Autodesk Inventor part; units mm, degrees
ref_plane "Work Plane1" through (0, 0, 0) normal (0, -0.9396926, -0.3420201) x (-1, 0, 0)
ref_plane "YZ Plane" through (0, 0, 0) normal (1, 0, 0) x (0, 1, 0)
ref_plane "XZ Plane" through (0, 0, 0) normal (0, 1, 0) x (-1, 0, 0)
sketch "Sketch2" plane through (0, 0, 0) normal (0, 1, 0) x (-1, 0, 0)
  line L0 (0, 0) -> (-7, 0)
  line L1 (-7, 0) -> (-7, -10)
  line L2 (-7, -10) -> (0, -10)
  line L3 (0, -10) -> (0, 0)
  circle A0 centre (-3.5, -5) radius 1.65
  line L4 (0, 0) -> (15, 0)
  line L5 (15, 0) -> (15, -15.9854)
  line L6 (15, -15.9854) -> (0, -15.9854)
  line L7 (0, -15.9854) -> (0, 0)
  line L8 (7.8, 0) -> (10.8, 0)
  line L9 (10.8, 0) -> (10.8, -15.9854)
  line L10 (10.8, -15.9854) -> (7.8, -15.9854)
  line L11 (7.8, -15.9854) -> (7.8, 0)
  line L12 (15, -15.9854) -> (10.8, -15.9854)
  line L13 (10.8, -15.9854) -> (10.8, -4.2527)
  line L14 (10.8, -4.2527) -> (15, -4.2527)
  line L15 (15, -4.2527) -> (15, -15.9854)
  line L16 (0, -10) -> (10.8, -10)
  point P0 (0, -5)
  point P1 (-3.5, -10)
  point P2 (10.8, 0)
  point P3 (15, -4.2527)
  point P4 (7.8, -10)
  dimension "d2" = 7
  dimension "d3" = 10
  dimension "d4" = 3.3
  dimension "d12" = 22
  dimension "d21" = 11.3
  dimension "d22" = 3
extrude "Extrusion1" add sketch "Sketch2" along normal blind 4.5 contours L3 L2 L1 L0
extrude "Extrusion2" add sketch "Sketch2" along normal blind 4 contours L4 L11 L16 L3 | L4 L9 L16 L11 | L4 L5 L14 L9
ref_plane "Work Plane1" through (0, 0, 0) normal (0, -0.9396926, -0.3420201) x (-1, 0, 0)
sketch "Sketch4" plane through (-15, 0, -15.9854) normal (-1, 0, 0) x (0, 0, 1)
  line L0 (-0.8784, 3) -> (12.8006, -3.1551)
  line L1 (12.8006, -3.1551) -> (13.2109, -2.2432)
  line L2 (13.2109, -2.2432) -> (-0.4681, 3.9119)
  line L3 (-0.8784, 3) -> (-0.4681, 3.9119)
  arc A0 (18.4229, -40.6351) -> (9.5813, -1.7065) centre (-0.6772, -24.5048) ccw
  line L4 (18.4229, -40.6351) -> (19.1869, -41.2803)
  line L5 (9.5813, -1.7065) -> (10.2986, -0.9327)
  arc A1 (19.1869, -41.2803) -> (10.2986, -0.9327) centre (-0.2668, -24.413) ccw
  arc A2 (18.4229, -40.6351) -> (17.1504, -48.2979) centre (24.2261, -45.5359) ccw
  arc A3 (19.1869, -41.2803) -> (18.0819, -47.9342) centre (24.064, -45.509) ccw
  line L6 (17.1504, -48.2979) -> (18.0819, -47.9342)
  line L7 (22.6596, -12.694) -> (22.6596, 0.6055)
  line L8 (22.6596, 0.6055) -> (12.4332, 0.6055)
  line L9 (12.4332, 0.6055) -> (12.4332, 1.6055)
  line L10 (12.4332, 1.6055) -> (23.6596, 1.6055)
  line L11 (23.6596, 1.6055) -> (23.6596, -14.9008)
  line L12 (5.9854, 0) -> (11.7327, 0)
  arc A4 (2.815, 4.6033) -> (3.1019, 1.209) centre (3.9014, 2.9858) ccw
  line L13 (2.815, 4.6033) -> (2.815, 3.6033)
  arc A5 (2.815, 3.6033) -> (3.0226, 2.3412) centre (3.3375, 3.0411) ccw
  point P0 (15.9854, 0)
  point P1 (13.4215, -1.7995)
  point P2 (1.9601, 2.8193)
  point P3 (2.654, 2.6401)
  dimension "d14" = 1
  dimension "d20" = 15
  dimension "d26" = 25
  dimension "d27" = 1
  dimension "d29" = 1
  dimension "d30" = 1
  dimension "d31" = 1
  dimension "d35" = 3
  dimension "d37" = 1
  dimension "d38" = 1
extrude "Extrusion4" add sketch "Sketch4" along normal blind 10 contours A4 L2 L5 L0 | L5 A1 L1 L0 | L0 L1 A1 L4 A0 | A4 L13 A5 L2 | L4 A3 L6 A2 | L7 L8 L9 L10 L11 A1
extrude "Extrusion5" add sketch "Sketch2" against normal blind 6 contours L4 L9 L16 L11
chamfer "Chamfer1" distance 2 angle 45 1 edges at (-15, 2, -4.2527)
properties part number "spool_blocker"
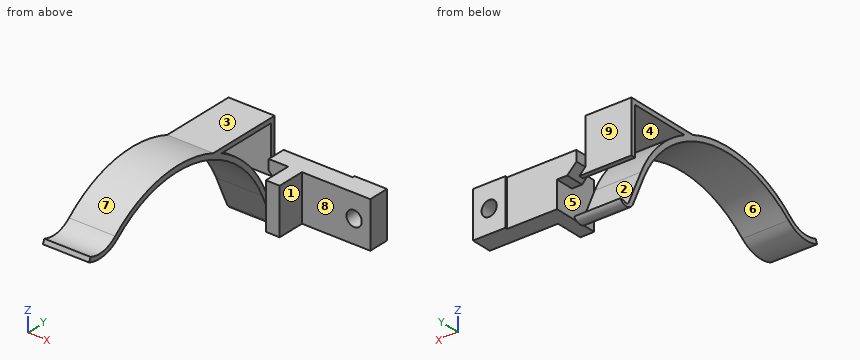
Work out the finished part from the listing and answer in its coordinate system (mm). Face numbers are marked on the shaded views. A direction names the side the tool comes from. Give positions to 0.01 mm unless a question says otherwise; leave off trailing zeros. Order: outer loops, then holes, each group sorted by start corner. A loop starts at its lowest first (then second) coordinate and runs counter-clockwise, first axis right, second up.
1. Each of these flat-tipped pins is pushed along its axis until it touches: P1, Ø10, axis at x = -6.5, z = -6.5, coming from the +Y side; P2, Ø3.5, axis at x = -8.5, z = -7, coming from the -Y side; P3, Ø11.5, axis at x = -3, y = -0.5, coming from the -Z side. Where does it stop, or does it pass through?
Result sheet:
P1: stops at y = 4
P2: stops at y = -6
P3: stops at z = -10
2. Section C-C, the plane y = -11.5 is taken. Determine the outline of the cut face in (x, z), and give its area (3 significant figures).
Result sheet:
outline: (-25, 4.69) - (-15, 4.69) - (-15, 6.02) - (-25, 6.02) - close; (-25, 6.67) - (-15, 6.67) - (-15, 7.67) - (-25, 7.67) - close
area: 23.3 mm2
3. For the marked faces 1, 2, 3, 4 and 5, determine the directions among +Z, -Z, +X, -X, +Y, -Y from which every point of the face is accessible in a straight line to the end or side of a thin tool.
Result sheet:
face 1: +Z, -Z, +X, -Y
face 2: -X, +Y
face 3: +Z, +X, -X, +Y
face 4: +X, -X
face 5: -Z, -Y
4. Section D-D, the plane x = -3.5 is taken. Determine the outline of the cut face in (y, z), and give its area (3 significant figures).
Result sheet:
outline: (0, -10) - (4, -10) - (4, 0) - (0, 0) - close
area: 40.0 mm2
5. Straight lines are drawn through the part: L1, parallel to Z at x = 3.5, y = 2.2; L2, parallel to Y at x = -5, z = -6.5; L3, parallel to Y at x = 1, z = -4. For each, find the intervals that lie inside material, in ascending order.
Result sheet:
L1: z = -10 to -6.65, -3.35 to 0
L2: y = 0 to 4
L3: y = 0 to 4.5
6. The mould has two halves that part along Y. Classify the marked faces 6, 7, 8 and 9: released by +Y, released by -Y, zero draft, split by the parting line, or undercut.
Result sheet:
face 6: undercut
face 7: split by the parting line
face 8: released by -Y
face 9: released by +Y
7. Section B-B, the plane z = -7.25 is taken. Determine the outline of the cut face in (x, y), and give its area (3 significant figures).
Result sheet:
outline: (-25, -1.33) - (-15, -1.33) - (-15, -0.23) - (-25, -0.23) - close; (-10.8, -6) - (-7.8, -6) - (-7.8, 0) - (7, 0) - (7, 4.5) - (0, 4.5) - (0, 4) - (-10.8, 4) - close
area: 104 mm2
8. Section A-A, the plane x = 3.5 is taken. Determine the outline of the cut face in (y, z), and give its area (4 significant figures).
Result sheet:
outline: (0, -10) - (4.5, -10) - (4.5, -6.65) - (0, -6.65) - close; (0, -3.35) - (4.5, -3.35) - (4.5, 0) - (0, 0) - close
area: 30.15 mm2
